Here's how the part is built. I have some questions about the finished solid (model axes, mm). Face numbers are marked on the shaded views. A direction names the side the tool comes from. Give positions to 0.01 mm unless a question says otherwise; leave off trailing zeros. Loops run counter-clockwise (first coordinate to the right, second up) from the corner with the lowest first, then second, coordinate; pieces in that order, holes last. Notation, with made-up numbers: (-0.75, -39) - (47.25, -39) arc R23 cw to (47.25, -15) - close; hole circle Ø3 at (70, 43). An arc over 180 degrees is marked (long way). Use a Markdown table: item, result.
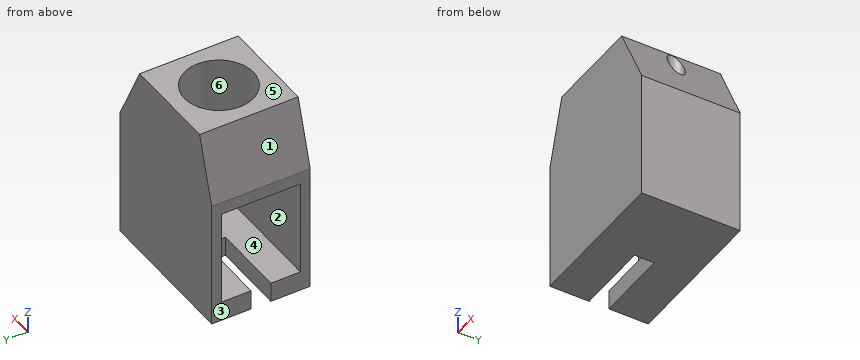
from build123d import *

# Parameters (mm, degrees)
PAD001_DEPTH    = 2.5
SKETCH003_W     = 1
SKETCH003_H     = 1
POCKET_DEPTH    = 3.75
SKETCH004_W     = 4.87
SKETCH004_H     = 4
POCKET001_DEPTH = 6.8
SKETCH005_R     = 1.75
SKETCH005_R_2   = 0.4
POCKET002_DEPTH = 5


with BuildPart() as part:
    # Sketch002 → Pad001 (new body, symmetric)
    with BuildSketch(Plane.XZ):
        Polygon((0, 0), (7.6, 0), (7.6, 6.5), (5.95, 9.8), (1, 9.8), (0, 6.5), align=None)
    extrude(amount=PAD001_DEPTH, both=True)

    # Sketch003 (on Face6 of Pad001) → Pocket (cut)
    with BuildSketch(Plane(origin=(0, 0, 0), x_dir=(0, 0, -1), z_dir=(-1, 0, 0))):
        with Locations((-0.5, 0)):
            Rectangle(SKETCH003_W, SKETCH003_H)
    extrude(amount=-POCKET_DEPTH, mode=Mode.SUBTRACT)

    # Sketch004 (on Face5 of Pocket) → Pocket001 (cut)
    with BuildSketch(Plane(origin=(0, 0, 0), x_dir=(0, 0, -1), z_dir=(-1, 0, 0))):
        with Locations((-3.435, 0)):
            Rectangle(SKETCH004_W, SKETCH004_H)
    extrude(amount=-POCKET001_DEPTH, mode=Mode.SUBTRACT)

    # Sketch005 (on Face10 of Pocket001) → Pocket002 (cut)
    with BuildSketch(Plane(origin=(0, 0, 9.8), x_dir=(-1, 0, 0), z_dir=(0, 0, 1))):
        with Locations((-3.475, 0)):
            Circle(SKETCH005_R)
        with Locations((-6.375, 0)):
            Circle(SKETCH005_R_2)
    extrude(amount=-POCKET002_DEPTH, mode=Mode.SUBTRACT)


solid = part.part
(1) Will this pin go through, and if not, where does the flat tip stop? pin 1 (1.2 mm diameter, centred on y = 0.5, z = 3.5, fed in from -X).
A:
| item | result |
|---|---|
| pin 1 | x = 6.8 |
(2) Suppose I cut it at A-A on y = 0. Write out the boundary of the cut face in (x, z) (3 decimals), plus the area to 3 significant figures.
A:
| item | result |
|---|---|
| outline | (0, 5.87) - (1.725, 5.87) - (1.725, 9.8) - (1, 9.8) - (0, 6.5) - close; (3.75, 0) - (7.6, 0) - (7.6, 6.5) - (6.775, 8.15) - (6.775, 5.87) - (6.8, 5.87) - (6.8, 1) - (3.75, 1) - close; (5.225, 5.87) - (5.975, 5.87) - (5.975, 9.75) - (5.95, 9.8) - (5.225, 9.8) - close |
| area | 17.0 mm2 |
(3) We'd pull the mould along Z, two halves only. Please class the marked faces 1, 2 and 3: pulls with the +Z half, pulls with the -Z half, needs draft (parallel to the pull), parting line crosses it, or undercut.
A:
| item | result |
|---|---|
| face 1 | pulls with the +Z half |
| face 2 | undercut |
| face 3 | needs draft |
(4) Suppose I cut it at C-C on z = 6. Write out the boundary of the cut face in (x, y) (3 decimals).
A:
| item | result |
|---|---|
| outline | (0, -2.5) - (7.6, -2.5) - (7.6, 2.5) - (0, 2.5) - close; hole circle Ø3.5 at (3.475, 0); hole circle Ø0.8 at (6.375, 0) |
(5) If I drill on line 1 (Y direction, x = 0.5, z = 4.75); line 2 (Z direction, x = 1.5, y = 1.2); line 3 (X direction, y = 0, z = 7) (3 decimals), over which ranges is the centre line in solid material (lowest first)?
A:
| item | result |
|---|---|
| line 1 | -2.5 to -2, 2 to 2.5 |
| line 2 | 0 to 1, 5.87 to 9.8 |
| line 3 | 0.152 to 1.725, 5.225 to 5.975, 6.775 to 7.35 |
(6) Suppose I cut it at B-B on x = 1.25. Write out the boundary of the cut face in (y, z), plus the area to 3 significant figures.
A:
| item | result |
|---|---|
| outline | (-2.5, 0) - (-0.5, 0) - (-0.5, 1) - (-2, 1) - (-2, 5.87) - (2, 5.87) - (2, 1) - (0.5, 1) - (0.5, 0) - (2.5, 0) - (2.5, 9.8) - (-2.5, 9.8) - close |
| area | 28.5 mm2 |
(7) On a 3-axis mill with a long thin cutter (end or side, diameter ignored), from which of +Z, -Z, +X, -X, +Y, -Y can I reach the whole of each face in a straight line? I mean the marked faces 4, 5 and 6. Say none if no direction works.
A:
| item | result |
|---|---|
| face 4 | -X |
| face 5 | +Z, +X, -X, +Y, -Y |
| face 6 | +Z |
(8) Suppose I cut it at D-D on y = 0.75. Write out the boundary of the cut face in (x, z), plus the area to 3 significant figures.
A:
| item | result |
|---|---|
| outline | (0, 0) - (7.6, 0) - (7.6, 6.5) - (5.95, 9.8) - (5.06, 9.8) - (5.06, 5.87) - (6.8, 5.87) - (6.8, 1) - (0, 1) - close; (0, 5.87) - (1.89, 5.87) - (1.89, 9.8) - (1, 9.8) - (0, 6.5) - close |
| area | 24.6 mm2 |
